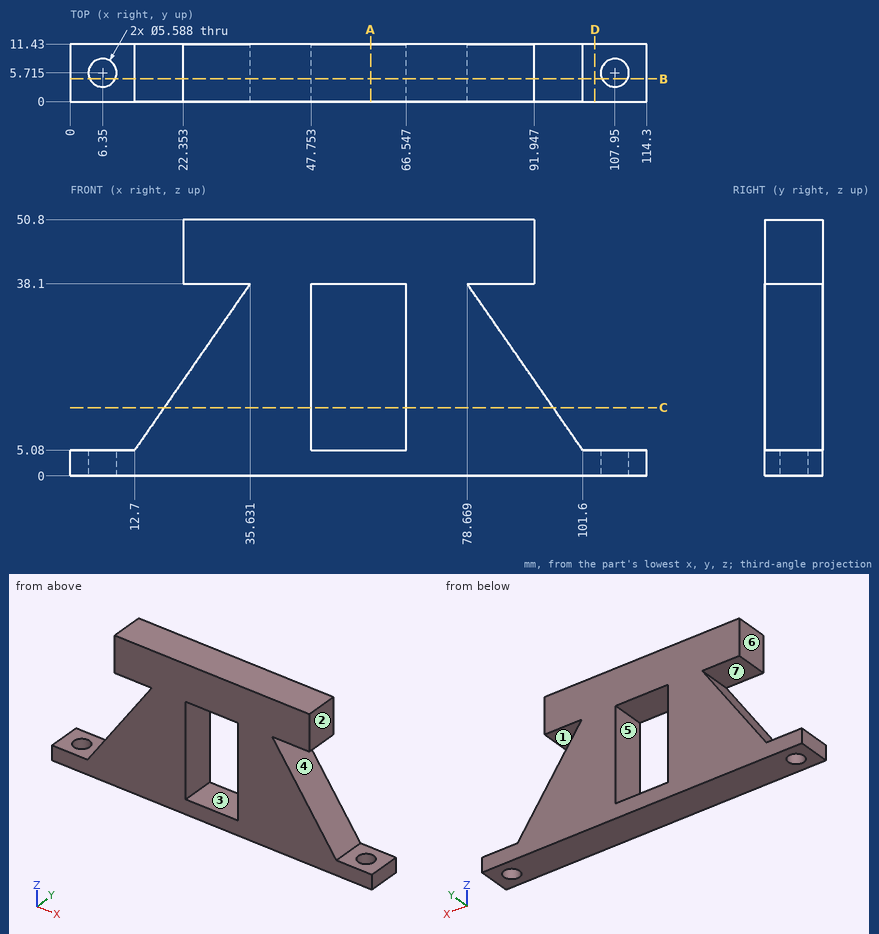
Job drawing, mm, ordinate dimensions from the low corner. One solid piece. A direction names the side the tool comes from. Give positions to 0.01 mm unless a question says otherwise; leave off trailing zeros. Order: outer loops, then holes, each group sorted by start corner. A loop starts at its lowest first (then second) coordinate and runs counter-clockwise, first axis right, second up. Notation, with made-up numbers: (-17.5, -18) - (1.5, -18) arc R20 ccw to (1.5, -3) - close; hole circle Ø11 at (40, -13.75). An arc over 180 degrees is marked (long way). Return JSON: item names as keys, results as strings.
1) Cut at A-A, the plane x = 59.5. Give the cut face in (y, z), plus the area to 3 significant figures.
Geometry says:
{"outline": "(0, 0) - (11.43, 0) - (11.43, 5.08) - (0, 5.08) - close; (0, 38.1) - (11.43, 38.1) - (11.43, 50.8) - (0, 50.8) - close", "area": "203 mm²"}
2) Pull direction X, two halves, no side cores. Call the marked faces 1, 2 and 3: pulls with the +X half, pulls with the -X half, needs draft (parallel to the pull), parting line crosses it, or undercut.
Geometry says:
{"face 1": "needs draft", "face 2": "pulls with the +X half", "face 3": "undercut"}
3) 3-axis set-ups, long thin cutter, end or side, ignore diameter. For the marked faces 4, 5, 6 and 7: which of +Z, -Z, +X, -X, +Y, -Y reach the whole face in a straight line?
Geometry says:
{"face 4": "+X, +Y, -Y", "face 5": "+Y, -Y", "face 6": "+Z, -X, +Y, -Y", "face 7": "-X, +Y, -Y"}
4) Cut at C-C, the plane z = 13.5. Give the cut face in (x, y).
Geometry says:
{"outline": "(18.55, 0) - (47.75, 0) - (47.75, 11.43) - (18.55, 11.43) - close; (66.55, 0) - (95.75, 0) - (95.75, 11.43) - (66.55, 11.43) - close"}
5) Flat gauge pins, fed straight in: P1, Ø3.5, axis at y = 5, z = 46.5, coming from the -X side; P2, Ø4, axis at y = 7.5, z = 17, coming from the -X side; P3, Ø6.5, axis at x = 6.35, y = 5.715, coming from the +Z side; P4, Ø3.5, axis at x = 107.95, y = 5.715, coming from the -Z side. Where does each tip first touch, or does it go through?
Geometry says:
{"P1": "x = 22.35", "P2": "x = 19.59", "P3": "z = 5.08", "P4": "through"}
6) Probe line 1 (Y direction, x = 6.35, z = 2.8); line 2 (Z direction, x = 102.5, y = 6.5); line 3 (Z direction, x = 25, y = 4.25) (1 decimal). List the from-to ranges inside material, lowest first. Write a range as from..to.
Geometry says:
{"line 1": "0..2.92, 8.51..11.43", "line 2": "0..5.08", "line 3": "0..22.8, 38.1..50.8"}
7) Cut at D-D, the plane x = 104. Give the cut face in (y, z).
Geometry says:
{"outline": "(0, 0) - (11.43, 0) - (11.43, 5.08) - (0, 5.08) - close"}
8) Cut at B-B, the plane y = 4.5. Give the cut face in (x, z).
Geometry says:
{"outline": "(0, 0) - (3.83, 0) - (3.83, 5.08) - (0, 5.08) - close; (8.87, 0) - (105.43, 0) - (105.43, 5.08) - (101.6, 5.08) - (78.67, 38.1) - (91.95, 38.1) - (91.95, 50.8) - (22.35, 50.8) - (22.35, 38.1) - (35.63, 38.1) - (12.7, 5.08) - (8.87, 5.08) - close; (110.47, 0) - (114.3, 0) - (114.3, 5.08) - (110.47, 5.08) - close; hole (47.75, 5.08) - (66.55, 5.08) - (66.55, 38.1) - (47.75, 38.1) - close"}
